Source: CAD feature listing. Evaluate the final solid. Frame: model axes, mm. A direction names the side the tool comes from. Give positions to 0.01 mm unless a question says otherwise; leave off trailing zeros. Loops run counter-clockwise (first coordinate to the right, second up) from the corner with the lowest first, then second, coordinate; pieces in that order, holes last. Notation, with made-up numbers: (-7, 77.5) -> (47, 77.5) arc R27 cw to (47, 106.5) -> close; hole circle Ø8 at (49.25, -20.5). An arc over 180 degrees is marked (long way). Return JSON: item names as keys, results as strings. Group by question number.
Autodesk Inventor part; units mm, degrees
ref_plane "YZ Plane" through (0, 0, 0) normal (1, 0, 0) x (0, 1, 0)
ref_plane "XZ Plane" through (0, 0, 0) normal (0, 1, 0) x (-1, 0, 0)
ref_plane "XY Plane" through (0, 0, 0) normal (0, 0, 1) x (1, 0, 0)
sketch "Sketch1" plane through (0, 0, 0) normal (0, 1, 0) x (-1, 0, 0)
  line L0 (100, -50) -> (-100, -50)
  line L1 (-100, -50) -> (-100, 50)
  line L2 (-100, 50) -> (100, 50)
  line L3 (100, 50) -> (100, -50)
  line L4 (100, -50) -> (-100, 50) construction
  line L5 (-100, -50) -> (100, 50) construction
  line L6 (-40, -30) -> (-80, -30)
  line L7 (-50, -50) -> (-70, -50)
  line L8 (-40, -30) -> (-50, -50)
  line L9 (-80, -30) -> (-70, -50)
  line L10 (80, -30) -> (40, -30)
  line L11 (70, -50) -> (50, -50)
  line L12 (80, -30) -> (70, -50)
  line L13 (40, -30) -> (50, -50)
  line L14 (-100, -10) -> (-100, 10)
  line L15 (-80, -20) -> (-80, 20)
  line L16 (-80, -20) -> (-100, -10)
  line L17 (-80, 20) -> (-100, 10)
  point P0 (0, 0)
  point P1 (-100, 10)
  point P2 (-100, -10)
  point P3 (-70, -50)
  point P4 (-50, -50)
  point P5 (70, -50)
  point P6 (0, 0)
  point P7 (0, 0)
  dimension "d72" = 200
  dimension "d73" = 100
  dimension "d78" = 20
  dimension "d79" = 40
  dimension "d80" = 20
  dimension "d81" = 10
  dimension "d82" = 20
  dimension "d83" = 40
  dimension "d84" = 20
  dimension "d85" = 10
  dimension "d86" = 120
  dimension "d87" = 30
  dimension "d88" = 0
  dimension "d89" = 0
  dimension "d90" = 40
  dimension "d91" = 20
  dimension "d92" = 20
  dimension "d93" = 10
  dimension "d94" = 40
  dimension "d95" = 0
extrude "Extrusion17" add sketch "Sketch1" along normal blind 10
extrude "Extrusion18" cut sketch "Sketch1" along normal blind 6 contours L0 L13 L10 L12 | L0 L9 L6 L8 | L17 L15 L16 L1
pattern_circular "Circular Pattern5" count 2 over 360 about axis through (0, -10, 0) along (0, 1, 0) of "Extrusion18"
fillet "Fillet6" radius 2 12 edges at (80, 3, -30) (40, 3, -30) (-40, 3, -30) (-80, 3, -30) (-80, 3, -20) (-80, 3, 20) (-80, 3, 30) (-40, 3, 30) (40, 3, 30) (80, 3, 30) (80, 3, 20) (80, 3, -20)
sketch "Sketch5" plane through (0, 10, 0) normal (0, 1, 0) x (1, 0, 0)
  line L0 (100, -50) -> (100, -10)
  line L1 (100, 50) -> (-100, 50)
  line L2 (100, -50) -> (0, -50)
  line L3 (0, -50) -> (0, 50)
  line L4 (0, 50) -> (100, 50)
  line L5 (100, 50) -> (100, -50)
  point P0 (0, 0)
extrude "Extrusion19" add sketch "Sketch5" along normal blind 2
properties part number "Test2_3DPrint"
1) Cut plane C-C on z = 37.5. Return loops of the section in (x, y).
2) Reachability of faces 1 (the face through (60, 3, 30)), 2 (the face through (1, 6, -50)) from +Z, -Z, +X, -X, +Y, -Y: full face, straight path, thin tool, end or side. Return the list, or none.
3) Cut plane B-B on x = 61. Return loops of the section in (y, z).
4) Cut plane D-D on x = -45.5. Return loops of the section in (y, z).
5) Cut plane A-A on z = 4. Return loops of the section in (x, y).
6) Contact query for flat-ended pins moving along their axis: P1, Ø1, axis at y = 11, z = 1.5, coming from the -X side; P2, Ø3, axis at x = -62.5, y = 4, coming from the +Z side; P3, Ø3, axis at x = -56.5, y = 4, coming from the -Z side. Output: stop coordinate, or through.
7) Material intervals for line 1 (X direction, y = 5.25, z = -13.5); line 2 (Y direction, x = -59, z = 16.5); line 3 (X direction, y = 4.75, z = -43), sorted ascending.
8) Mould query, pull axis Z, two halves, no side actions, for faces 3 (the face through (-74.336, 2.958, -41.327)), 4 (the face through (100, 7, 1)), 5 (the face through (1, 6, 50)). Classes: released by +Z, released by -Z, zero draft, split by the parting line, or undercut.
Calculated:
{
 "1": {"outline": "(-100, 0) -> (-76.25, 0) -> (-76.25, 6) -> (-43.75, 6) -> (-43.75, 0) -> (43.75, 0) -> (43.75, 6) -> (76.25, 6) -> (76.25, 0) -> (100, 0) -> (100, 12) -> (0, 12) -> (0, 10) -> (-100, 10) -> close"},
 "2": {"face 1": "-Y", "face 2": "-Z, +X, -X, +Y, -Y"},
 "3": {"outline": "(0, -30) -> (6, -30) -> (6, -50) -> (12, -50) -> (12, 50) -> (6, 50) -> (6, 30) -> (0, 30) -> close"},
 "4": {"outline": "(0, -50) -> (10, -50) -> (10, 50) -> (0, 50) -> (0, 41) -> (6, 41) -> (6, 30) -> (0, 30) -> (0, -30) -> (6, -30) -> (6, -41) -> (0, -41) -> close"},
 "5": {"outline": "(-100, 6) -> (-80, 6) -> (-80, 0) -> (80, 0) -> (80, 6) -> (100, 6) -> (100, 12) -> (0, 12) -> (0, 10) -> (-100, 10) -> close"},
 "6": {"P1": "x = 0", "P2": "z = 30", "P3": "z = -30"},
 "7": {"line 1": "-100 to -93, -80 to 80, 93 to 100", "line 2": "0 to 10", "line 3": "-100 to -73.5, -46.5 to 46.5, 73.5 to 100"},
 "8": {"face 3": "undercut", "face 4": "zero draft", "face 5": "released by +Z"}
}
